Geometry check sheet. Reference: the model listing, model coordinates, mm. Round coordinates to 2 decimals unless told otherwise and drop trailing zeros. Order: outer loops, then holes, each group sorted by start corner. A loop starts at its lowest first (then second) coordinate and runs counter-clockwise, first axis right, second up.
```python
from build123d import *

# Parameters (mm, degrees)
F1_DEPTH = 5
F2_R     = 2


with BuildPart() as f1:
    # F0 (on Top) → F1 (new body)
    with BuildSketch(Plane.XY):
        Polygon((16.937762, 10), (-30, 10), (-16.937762, -10), (30, -10), align=None)
    extrude(amount=F1_DEPTH)

    # F2
    f2_edges = [f1.edges().sort_by_distance(p)[0] for p in [
        (6.531119, -10, 5),
        (-23.468881, 0, 5),
        (-23.468881, 0, 0),
        (23.468881, 0, 5),
        (30, -10, 2.5),
        (16.937762, 10, 2.5),
        (23.468881, 0, 0),
        (6.531119, -10, 0),
        (-16.937762, -10, 2.5),
    ]]
    fillet(f2_edges, radius=F2_R)


solid = f1.part
```
(1) Sectioned sample at A-A, the plane x = 5.5. Record the cut outline in (y, z), and give its area (3 significant figures).
Returned:
outline: (-10, 2) arc R2 ccw to (-8, 0) - (10, 0) - (10, 5) - (-8, 5) arc R2 ccw to (-10, 3) - close
area: 98.3 mm2
(2) Depth check by flat-ended pin: P1, Ø2, axis at x = -19.5, z = 3.5, coming from the -Y side. Enter the tip coordinate at first touch or a pass-through.
Returned:
P1: stops at y = -7.54
(3) Sectioned sample at B-B, the plane z = 1.5. Record the cut outline in (x, y) (1 decimal).
Returned:
outline: (-29.9, 10) - (-17.5, -9.1) arc R1.9 ccw to (-15.9, -9.9) - (26.3, -9.9) arc R1.9 ccw to (27.9, -6.9) - (17.2, 9.5) arc R2 ccw to (15.9, 10) - close
(4) Material ranges on line 1 (Y direction, x = -2.5, z = 1.25); line 2 (X direction, y = -4.5, z = 1.45); line 3 (Y direction, x = -22, z = 3.95), recorded low to high.
Returned:
line 1: y = -9.85 to 10
line 2: x = -20.44 to 26.32
line 3: y = -1.81 to 10
